Check sheet for the modelled part. Datum: model origin and axes. Units: mm. A direction names the side the tool comes from. Round coordinates to 2 decimals unless told otherwise and drop trailing zeros. Loops run counter-clockwise (first coordinate to the right, second up) from the corner with the lowest first, then second, coordinate; pieces in that order, holes last. Notation, with made-up numbers: (61.5, 63.25) - (86.5, 63.25) arc R14 cw to (86.5, 83.25) - close; hole circle Ø11 at (31, 62.5). An arc over 180 degrees is marked (long way). Answer in a Markdown table with one row per item. Add a question column.
(1) Mould release check, pull along X, two halves, no side actions. Record for faces 1 (the cylindrical face through (83.97, 6.39, 10.56)), 2 (the cylindrical face through (18.708, 11.028, 12.681)), 3 (the flat face through (95.2, 6.4, 4)), 4 (the flat face through (66, 6, 15)): +X half, -X half, draft (parallel to the pull), parting line (faces both ways), or undercut.
(2) Cross-section at B-B on x = 95. Enter the section's corners in (y, z).
(3) Access from +Z, -Z, +X, -X, +Y, -Y to the whole of each face (thin tool, end or side, straight path). Record for faces 5 (the cylindrical face through (18.708, 2.028, 12.681)), 6 (the flat face through (134, 4, 0)), 7 (the flat face through (134, 9, 0)), 8 (the cylindrical face through (-15, 6, 0)), 9 (the flat face through (88, 6, 6)).
(4) Thickness scan on line 1 along Z through (x, y) = (106.5, 3.75); line 2 along X through (y, z) = (7.45, 0); line 3 along X through (y, z) = (7.25, 12). Record the ranges inside material, lowest first.
(5) Cross-section at C-C on z = -10.5. Enter the section's corners in (x, y).
(6) Gauge pin test, flat ends, axial feed: pin 1 (3.5 mm diameter, centred on x = 116, y = 7, fed in from +Z); pin 2 (1.2 mm diameter, centred on y = 3, z = -1, fed in from +X); pin 3 (4.5 mm diameter, centred on x = 134.5, z = -5, fed in from +Y). Record the tip position at first contact, or that the pin passes through.
(7) Cross-section at A-A on z = 3.5. Enter the section's corners in (x, y), then the cut area to 3 significant figures.
from build123d import *

# Parameters (mm, degrees)
MAIN_R              = 8
BOSS_EXTRUDE1_DEPTH = 13
CUT_EXTRUDE5_START  = -4
CUT_EXTRUDE5_DEPTH  = 4
CUT_EXTRUDE6_DEPTH  = 4
JOINT_HOLE_R        = 8.5
CUT_EXTRUDE7_DEPTH  = 13
CUT_EXTRUDE8_DEPTH  = 9
SKETCH9_R           = 20.014179858
CUT_EXTRUDE9_DEPTH  = 4
CUT_EXTRUDE10_START = -4
SKETCH10_R          = 20.014179858
CUT_EXTRUDE10_DEPTH = 4
FILLET1_R           = 5
FILLET2_R           = 5
CUT_EXTRUDE11_DEPTH = 5
CHAMFER1_START      = 3.94488544
CHAMFER1_DEPTH      = 5


with BuildPart() as part:
    # main → Boss-Extrude1 (new body)
    with BuildSketch(Plane(origin=(0, 0, 0), x_dir=(1, 0, 0), z_dir=(0, 1, 0))):
        with BuildLine():
            Line((0, 15), (130, 15))
            ThreePointArc((130, 15), (145, 0), (130, -15))
            Line((130, -15), (0, -15))
            ThreePointArc((0, -15), (-15, 0), (0, 15))
        make_face()
        with Locations(Location((0, 0, 0), (0, 0, 270))):
            Circle(MAIN_R, mode=Mode.SUBTRACT)
    extrude(amount=BOSS_EXTRUDE1_DEPTH)

    # Sketch5 → Cut-Extrude5 (cut)
    with BuildSketch(Plane(origin=(0, 13, 0), x_dir=(1, 0, 0), z_dir=(0, 1, 0)).offset(CUT_EXTRUDE5_START)):
        with BuildLine():
            Line((130, 15), (130, -15))
            ThreePointArc((130, -15), (145, 0), (130, 15))
        make_face()
    extrude(amount=CUT_EXTRUDE5_DEPTH, mode=Mode.SUBTRACT)

    # Sketch6 → Cut-Extrude6 (cut)
    with BuildSketch(Plane.XZ):
        with BuildLine():
            Line((130, 15), (130, -15))
            ThreePointArc((130, -15), (145, 0), (130, 15))
        make_face()
    extrude(amount=-CUT_EXTRUDE6_DEPTH, mode=Mode.SUBTRACT)

    # joint hole → Cut-Extrude7 (cut)
    with BuildSketch(Plane.XZ):
        with Locations(Location((106.49845917, 3.136605167, 0), (0, 0, 270))):
            Circle(JOINT_HOLE_R)
    extrude(amount=-CUT_EXTRUDE7_DEPTH, mode=Mode.SUBTRACT)

    # cut_out joint → Cut-Extrude8 (cut)
    with BuildSketch(Plane.XY.offset(15)):
        with BuildLine():
            Line((86.468116833, 8.94488544), (116.468116833, 8.94488544))
            ThreePointArc((116.468116833, 8.94488544), (118.968116833, 6.44488544), (116.468116833, 3.94488544))
            Line((116.468116833, 3.94488544), (86.468116833, 3.94488544))
            ThreePointArc((86.468116833, 3.94488544), (83.968116833, 6.44488544), (86.468116833, 8.94488544))
        make_face()
    extrude(amount=-CUT_EXTRUDE8_DEPTH, mode=Mode.SUBTRACT)

    # Sketch9 → Cut-Extrude9 (cut)
    with BuildSketch(Plane(origin=(0, 13, 0), x_dir=(1, 0, 0), z_dir=(0, 1, 0))):
        Circle(SKETCH9_R)
    extrude(amount=-CUT_EXTRUDE9_DEPTH, mode=Mode.SUBTRACT)

    # Sketch10 → Cut-Extrude10 (cut)
    with BuildSketch(Plane.XZ.offset(CUT_EXTRUDE10_START)):
        Circle(SKETCH10_R)
    extrude(amount=CUT_EXTRUDE10_DEPTH, mode=Mode.SUBTRACT)

    # Fillet1
    fillet1_edges = [part.edges().sort_by_distance(p)[0] for p in [
        (13.25018473, 2, 15),
    ]]
    fillet(fillet1_edges, radius=FILLET1_R)

    # Fillet2
    fillet2_edges = [part.edges().sort_by_distance(p)[0] for p in [
        (13.25018473, 11, 15),
    ]]
    fillet(fillet2_edges, radius=FILLET2_R)

    # Sketch11 → Cut-Extrude11 (cut)
    with BuildSketch(Plane(origin=(0, 9, 0), x_dir=(1, 0, 0), z_dir=(0, 1, 0))):
        with BuildLine():
            ThreePointArc((136.154229069, 1.81236628), (135, 0), (136.154229069, -1.81236628))
            Line((136.154229069, -1.81236628), (137, 0))
            Line((137, 0), (136.154229069, 1.81236628))
        make_face()
        with BuildLine():
            Line((137, 0), (136.154229069, -1.81236628))
            ThreePointArc((136.154229069, -1.81236628), (138.074350534, -1.686941294), (139, 0))
            ThreePointArc((139, 0), (138.074350534, 1.686941294), (136.154229069, 1.81236628))
            Line((136.154229069, 1.81236628), (137, 0))
        make_face()
    extrude(amount=-CUT_EXTRUDE11_DEPTH, mode=Mode.SUBTRACT)

    # Chamfer1: read off the stored shape, not the designer's step
    # Chamfer1 outline → Chamfer1 (cut)
    with BuildSketch(Plane(origin=(0, 0, 0), x_dir=(1, 0, 0), z_dir=(0, 1, 0)).offset(CHAMFER1_START)):
        with BuildLine():
            Line((98.059452794, -2.120154778), (92.162759821, -6))
            Line((92.162759821, -6), (98.495274177, -6))
            ThreePointArc((98.495274177, -6), (98.05158318, -4.085439196), (98.059452794, -2.120154778))
        make_face()
    extrude(amount=CHAMFER1_DEPTH, mode=Mode.SUBTRACT)


solid = part.part
Answers:
| question | item | result |
|---|---|---|
| 1 | face 1 | undercut |
| 1 | face 2 | -X half |
| 1 | face 3 | undercut |
| 1 | face 4 | draft |
| 2 | outline | (0, -15) - (13, -15) - (13, 15) - (8.94, 15) - (8.94, 4.13) - (3.94, 4.13) - (3.94, 15) - (0, 15) - close |
| 3 | face 5 | -X, -Y |
| 3 | face 6 | +Z, -Z, +X, -Y |
| 3 | face 7 | +Z, -Z, +X, +Y |
| 3 | face 8 | -X, +Y, -Y |
| 3 | face 9 | +Z |
| 4 | line 1 | z = -15 to -5.36, 11.64 to 15 |
| 4 | line 2 | x = -15 to -8, 8 to 98.6, 114.4 to 135, 139 to 145 |
| 4 | line 3 | x = -9 to 84.1, 118.83 to 139 |
| 5 | outline | (-10.71, 4) - (17.04, 4) - (17.04, 0) - (130, 0) - (130, 4) - (140.71, 4) - (140.71, 9) - (130, 9) - (130, 13) - (17.04, 13) - (17.04, 9) - (-10.71, 9) - close |
| 6 | pin 1 | stops at z = 6 |
| 6 | pin 2 | stops at x = 130 |
| 6 | pin 3 | stops at y = 9 |
| 7 | outline | (-14.59, 4) - (-7.19, 4) - (-7.19, 9) - (-14.59, 9) - close; (7.19, 4) - (19.71, 4) - (19.71, 0) - (98.01, 0) - (98.01, 3.94) - (95.96, 3.94) - (95.96, 8.94) - (98.01, 8.94) - (98.01, 13) - (19.71, 13) - (19.71, 9) - (7.19, 9) - close; (114.99, 0) - (130, 0) - (130, 4) - (144.59, 4) - (144.59, 9) - (130, 9) - (130, 13) - (114.99, 13) - close |
| 7 | area | 1,380 mm^2 |
